Verification items for the finished model (mm, model axes). A direction names the side the tool comes from. Round coordinates to 2 decimals unless told otherwise and drop trailing zeros. Write each loop counter-clockwise with the first axis right and the second up, starting at its lowest first coordinate (ties: lowest second). Pieces come first, ordered by that corner, then holes. Notation, with made-up numbers: M 46,-23 L 74,-23 A18 cw 74,-10 Z; hole C 76,87 d4. An arc over 180 degrees is marked long. One line per item, written item: value. Start each with the question number.
Item 1: Thickness scan on probe 1 along Y at (x, z) = (-25, 1.75); probe 2 along X at (y, z) = (17.25, 1.7); probe 3 along Y at (x, z) = (11, 1.65). Record the ranges inside material, lowest first. Write a range as from..to.
Item 2: Section check A-A, the plane x = 29. Record the cut outline in (y, z) (3 decimals), then the cut area to 3 significant figures.
Item 3: Draft check along Y on faces 3 (the face through (46.84, 20.16, 0.74)), 4 (the face through (43.363, 14.133, 1.685)), 5 (the face through (-3.4, 13.2, 1.875)). Enter one of: +Y half, -Y half, draft (parallel to the pull), parting line (faces both ways), or undercut.
Item 4: Tool access check on faces 1 (the face through (1.97, 5.78, 1.68)), 2 (the face through (-54.25, -3.58, 0.74)). Record the directions out of +Z, -Z, +X, -X, +Y, -Y that give a thin tool (end or side, any length) a straight path to the whole face; none if there is none.
Item 5: Section check B-B, the plane y = 6.75. Record the cut outline in (x, z) (3 decimals).
from build123d import *

# Parameters (mm, degrees)
SKETCH1_W             = 98.893995825
SKETCH1_H             = 21.421924981
BOSS_EXTRUDE1_DEPTH   = 1.5
SKETCH1_R             = 0.75
BOSS_EXTRUDE1_2_DEPTH = 1.5
BOSS_EXTRUDE1_3_DEPTH = 1.5
SKETCH1_9_R           = 0.75
BOSS_EXTRUDE2_DEPTH   = 1.875
SKETCH1_10_W          = 99.493995825
SKETCH1_10_H          = 22.021924981
SKETCH1_10_W_2        = 98.893995825
SKETCH1_10_H_2        = 21.421924981
BOSS_EXTRUDE3_DEPTH   = 1.875
SKETCH1_11_W          = 99.493995825
SKETCH1_11_H          = 22.021924981
BOSS_EXTRUDE4_DEPTH   = 1.5


with BuildPart() as part:
    # Sketch1 → Boss-Extrude1 (new body)
    with BuildSketch(Plane.XY):
        with Locations((-3.702524559, 8.286725718)):
            Rectangle(SKETCH1_W, SKETCH1_H)
        with BuildLine():
            ThreePointArc((2.011897659, 12.737688209), (2.099765624, 12.949820243), (2.311897659, 13.037688209))
            Line((2.311897659, 13.037688209), (30.614473354, 13.037688209))
            ThreePointArc((30.614473354, 13.037688209), (31.364473354, 12.787688209), (32.114473354, 13.037688209))
            Line((32.114473354, 13.037688209), (38.573185506, 13.037688209))
            ThreePointArc((38.573185506, 13.037688209), (43.364473354, 14.037688209), (38.573185506, 15.037688209))
            Line((38.573185506, 15.037688209), (32.114473354, 15.037688209))
            ThreePointArc((32.114473354, 15.037688209), (31.364473354, 15.287688209), (30.614473354, 15.037688209))
            Line((30.614473354, 15.037688209), (-45.846814494, 15.037688209))
            ThreePointArc((-45.846814494, 15.037688209), (-50.638102341, 14.037688209), (-45.846814494, 13.037688209))
            Line((-45.846814494, 13.037688209), (-20.588102341, 13.037688209))
            ThreePointArc((-20.588102341, 13.037688209), (-20.375970307, 12.949820243), (-20.288102341, 12.737688209))
            Line((-20.288102341, 12.737688209), (-20.288102341, 10.774606087))
            ThreePointArc((-20.288102341, 10.774606087), (-20.138102341, 5.779110144), (-19.988102341, 10.774606087))
            Line((-19.988102341, 10.774606087), (-19.988102341, 12.737688209))
            ThreePointArc((-19.988102341, 12.737688209), (-19.900234376, 12.949820243), (-19.688102341, 13.037688209))
            Line((-19.688102341, 13.037688209), (1.411897659, 13.037688209))
            ThreePointArc((1.411897659, 13.037688209), (1.624029693, 12.949820243), (1.711897659, 12.737688209))
            Line((1.711897659, 12.737688209), (1.711897659, 10.774606087))
            ThreePointArc((1.711897659, 10.774606087), (1.861897659, 5.779110144), (2.011897659, 10.774606087))
            Line((2.011897659, 10.774606087), (2.011897659, 12.737688209))
        make_face(mode=Mode.SUBTRACT)
        with BuildLine():
            Line((13.014473354, 3.832527843), (13.014473354, 5.795609965))
            ThreePointArc((13.014473354, 5.795609965), (12.864473354, 10.791105907), (12.714473354, 5.795609965))
            Line((12.714473354, 5.795609965), (12.714473354, 3.832527843))
            ThreePointArc((12.714473354, 3.832527843), (12.626605388, 3.620395809), (12.414473354, 3.532527843))
            Line((12.414473354, 3.532527843), (-8.685526646, 3.532527843))
            ThreePointArc((-8.685526646, 3.532527843), (-8.897658681, 3.620395809), (-8.985526646, 3.832527843))
            Line((-8.985526646, 3.832527843), (-8.985526646, 5.795609965))
            ThreePointArc((-8.985526646, 5.795609965), (-9.135526646, 10.791105907), (-9.285526646, 5.795609965))
            Line((-9.285526646, 5.795609965), (-9.285526646, 3.832527843))
            ThreePointArc((-9.285526646, 3.832527843), (-9.373394612, 3.620395809), (-9.585526646, 3.532527843))
            Line((-9.585526646, 3.532527843), (-37.888102341, 3.532527843))
            ThreePointArc((-37.888102341, 3.532527843), (-38.638102341, 3.782527843), (-39.388102341, 3.532527843))
            Line((-39.388102341, 3.532527843), (-45.846814494, 3.532527843))
            ThreePointArc((-45.846814494, 3.532527843), (-50.638102341, 2.532527843), (-45.846814494, 1.532527843))
            Line((-45.846814494, 1.532527843), (-39.388102341, 1.532527843))
            ThreePointArc((-39.388102341, 1.532527843), (-38.638102341, 1.282527843), (-37.888102341, 1.532527843))
            Line((-37.888102341, 1.532527843), (38.573185506, 1.532527843))
            ThreePointArc((38.573185506, 1.532527843), (43.364473354, 2.532527843), (38.573185506, 3.532527843))
            Line((38.573185506, 3.532527843), (13.314473354, 3.532527843))
            ThreePointArc((13.314473354, 3.532527843), (13.102341319, 3.620395809), (13.014473354, 3.832527843))
        make_face(mode=Mode.SUBTRACT)
    extrude(amount=BOSS_EXTRUDE1_DEPTH)



with BuildPart() as body_2:
    # Sketch1 → Boss-Extrude1 2 (new body)
    with BuildSketch(Plane.XY):
        with Locations((31.364473354, 14.037688209)):
            Circle(SKETCH1_R)
    extrude(amount=BOSS_EXTRUDE1_2_DEPTH)


with BuildPart() as body_3:
    # Sketch1 → Boss-Extrude1 3 (new body)
    with BuildSketch(Plane.XY):
        with Locations((-38.638102341, 2.532527843)):
            Circle(SKETCH1_R)
    extrude(amount=BOSS_EXTRUDE1_3_DEPTH)


with BuildPart() as part_1:
    add(part.part)

    add(body_2.part)  # Boss-Extrude2 merges body 2

    add(body_3.part)  # Boss-Extrude2 merges body 3
    # Sketch1_9 → Boss-Extrude2 (add)
    with BuildSketch(Plane.XY):
        with BuildLine():
            Line((2.011897659, 12.737688209), (2.011897659, 10.774606087))
            ThreePointArc((2.011897659, 10.774606087), (1.861897659, 5.779110144), (1.711897659, 10.774606087))
            Line((1.711897659, 10.774606087), (1.711897659, 12.737688209))
            ThreePointArc((1.711897659, 12.737688209), (1.624029693, 12.949820243), (1.411897659, 13.037688209))
            Line((1.411897659, 13.037688209), (-19.688102341, 13.037688209))
            ThreePointArc((-19.688102341, 13.037688209), (-19.900234376, 12.949820243), (-19.988102341, 12.737688209))
            Line((-19.988102341, 12.737688209), (-19.988102341, 10.774606087))
            ThreePointArc((-19.988102341, 10.774606087), (-20.138102341, 5.779110144), (-20.288102341, 10.774606087))
            Line((-20.288102341, 10.774606087), (-20.288102341, 12.737688209))
            ThreePointArc((-20.288102341, 12.737688209), (-20.375970307, 12.949820243), (-20.588102341, 13.037688209))
            Line((-20.588102341, 13.037688209), (-45.846814494, 13.037688209))
            ThreePointArc((-45.846814494, 13.037688209), (-50.638102341, 14.037688209), (-45.846814494, 15.037688209))
            Line((-45.846814494, 15.037688209), (30.614473354, 15.037688209))
            ThreePointArc((30.614473354, 15.037688209), (31.364473354, 15.287688209), (32.114473354, 15.037688209))
            Line((32.114473354, 15.037688209), (38.573185506, 15.037688209))
            ThreePointArc((38.573185506, 15.037688209), (43.364473354, 14.037688209), (38.573185506, 13.037688209))
            Line((38.573185506, 13.037688209), (32.114473354, 13.037688209))
            ThreePointArc((32.114473354, 13.037688209), (31.364473354, 12.787688209), (30.614473354, 13.037688209))
            Line((30.614473354, 13.037688209), (2.311897659, 13.037688209))
            ThreePointArc((2.311897659, 13.037688209), (2.099765624, 12.949820243), (2.011897659, 12.737688209))
        make_face()
        with Locations((31.364473354, 14.037688209)):
            Circle(SKETCH1_9_R, mode=Mode.SUBTRACT)
        with BuildLine():
            ThreePointArc((13.014473354, 3.832527843), (13.102341319, 3.620395809), (13.314473354, 3.532527843))
            Line((13.314473354, 3.532527843), (38.573185506, 3.532527843))
            ThreePointArc((38.573185506, 3.532527843), (43.364473354, 2.532527843), (38.573185506, 1.532527843))
            Line((38.573185506, 1.532527843), (-37.888102341, 1.532527843))
            ThreePointArc((-37.888102341, 1.532527843), (-38.638102341, 1.282527843), (-39.388102341, 1.532527843))
            Line((-39.388102341, 1.532527843), (-45.846814494, 1.532527843))
            ThreePointArc((-45.846814494, 1.532527843), (-50.638102341, 2.532527843), (-45.846814494, 3.532527843))
            Line((-45.846814494, 3.532527843), (-39.388102341, 3.532527843))
            ThreePointArc((-39.388102341, 3.532527843), (-38.638102341, 3.782527843), (-37.888102341, 3.532527843))
            Line((-37.888102341, 3.532527843), (-9.585526646, 3.532527843))
            ThreePointArc((-9.585526646, 3.532527843), (-9.373394612, 3.620395809), (-9.285526646, 3.832527843))
            Line((-9.285526646, 3.832527843), (-9.285526646, 5.795609965))
            ThreePointArc((-9.285526646, 5.795609965), (-9.135526646, 10.791105907), (-8.985526646, 5.795609965))
            Line((-8.985526646, 5.795609965), (-8.985526646, 3.832527843))
            ThreePointArc((-8.985526646, 3.832527843), (-8.897658681, 3.620395809), (-8.685526646, 3.532527843))
            Line((-8.685526646, 3.532527843), (12.414473354, 3.532527843))
            ThreePointArc((12.414473354, 3.532527843), (12.626605388, 3.620395809), (12.714473354, 3.832527843))
            Line((12.714473354, 3.832527843), (12.714473354, 5.795609965))
            ThreePointArc((12.714473354, 5.795609965), (12.864473354, 10.791105907), (13.014473354, 5.795609965))
            Line((13.014473354, 5.795609965), (13.014473354, 3.832527843))
        make_face()
        with Locations((-38.638102341, 2.532527843)):
            Circle(SKETCH1_9_R, mode=Mode.SUBTRACT)
    extrude(amount=BOSS_EXTRUDE2_DEPTH)

    # Sketch1_10 → Boss-Extrude3 (add)
    with BuildSketch(Plane.XY):
        with Locations((-3.702524558, 8.286725718)):
            Rectangle(SKETCH1_10_W, SKETCH1_10_H)
        with Locations((-3.702524559, 8.286725718)):
            Rectangle(SKETCH1_10_W_2, SKETCH1_10_H_2, mode=Mode.SUBTRACT)
    extrude(amount=BOSS_EXTRUDE3_DEPTH)

    # Sketch1_11 → Boss-Extrude4 (add)
    with BuildSketch(Plane.XY):
        with BuildLine():
            ThreePointArc((-55.449522471, 17.297688209), (-54.277949596, 20.126115333), (-51.449522471, 21.297688209))
            Line((-51.449522471, 21.297688209), (44.044473354, 21.297688209))
            ThreePointArc((44.044473354, 21.297688209), (46.872900478, 20.126115333), (48.044473354, 17.297688209))
            Line((48.044473354, 17.297688209), (48.044473354, -0.724236772))
            ThreePointArc((48.044473354, -0.724236772), (46.872900478, -3.552663897), (44.044473354, -4.724236772))
            Line((44.044473354, -4.724236772), (-51.449522471, -4.724236772))
            ThreePointArc((-51.449522471, -4.724236772), (-54.277949596, -3.552663897), (-55.449522471, -0.724236772))
            Line((-55.449522471, -0.724236772), (-55.449522471, 17.297688209))
        make_face()
        with Locations((-3.702524558, 8.286725718)):
            Rectangle(SKETCH1_11_W, SKETCH1_11_H, mode=Mode.SUBTRACT)
    extrude(amount=BOSS_EXTRUDE4_DEPTH)


solid = part_1.part
Response values:
1. probe 1: y = -2.72..-2.42, 1.53..3.53, 13.04..15.04, 19..19.3
1. probe 2: x = -53.45..-53.15, 45.74..46.04
1. probe 3: y = -2.72..-2.42, 1.53..3.53, 6.63..9.96, 13.04..15.04, 19..19.3
2. outline: M -4.724,0 L 21.298,0 L 21.298,1.5 L 19.298,1.5 L 19.298,1.875 L 18.998,1.875 L 18.998,1.5 L 15.038,1.5 L 15.038,1.875 L 13.038,1.875 L 13.038,1.5 L 3.533,1.5 L 3.533,1.875 L 1.533,1.875 L 1.533,1.5 L -2.424,1.5 L -2.424,1.875 L -2.724,1.875 L -2.724,1.5 L -4.724,1.5 Z
2. area: 40.8 mm2
3. face 3: +Y half
3. face 4: undercut
3. face 5: draft
4. face 1: +Z
4. face 2: +Z, -Z, -X, -Y
5. outline: M -55.45,0 L 48.044,0 L 48.044,1.5 L 46.044,1.5 L 46.044,1.875 L 45.744,1.875 L 45.744,1.5 L 14.833,1.5 L 14.833,1.875 L 10.896,1.875 L 10.896,1.5 L 3.84,1.5 L 3.84,1.875 L -0.116,1.875 L -0.116,1.5 L -7.167,1.5 L -7.167,1.875 L -11.104,1.875 L -11.104,1.5 L -18.16,1.5 L -18.16,1.875 L -22.116,1.875 L -22.116,1.5 L -53.15,1.5 L -53.15,1.875 L -53.45,1.875 L -53.45,1.5 L -55.45,1.5 Z
